from build123d import *

# Parameters (mm, degrees)
EXTRUDE_START               = 15.8125
EXTRUDE_1_OUTLINE_W         = 35.35
EXTRUDE_1_OUTLINE_H         = 28.3375
EXTRUDE_1_DEPTH             = 9.5875
SKETCH_2_W                  = 35.35
SKETCH_2_H                  = 12.7
EXTRUDE_2_DEPTH             = 15.8125
SKETCH_3_W                  = 48.05
SKETCH_3_H                  = 25.4
EXTRUDE_3_DEPTH             = 6.35
SKETCH_4_W                  = 5.925
SKETCH_4_H                  = 6.096
EXTRUDE_4_DEPTH             = 11.5
SKETCH_5_W                  = 5.925
SKETCH_5_H                  = 6.096
EXTRUDE_5_DEPTH             = 11.5
HOLE_WIZARD_1_D             = 3.6576
HOLE_WIZARD_1_DEPTH         = 46.1875
HOLE_WIZARD_2_D             = 3.6576
HOLE_WIZARD_M8_1_D          = 9.525
HOLE_WIZARD_3_D             = 12.7
HOLE_WIZARD_M1_6_1_D        = 1.778
HOLE_WIZARD_M1_6_1_DEPTH    = 6.440714286
HOLE_WIZARD_M1_6_1_TIP      = 0.53416509
HOLE_WIZARD_1_7_1_7_1_D     = 1.7
HOLE_WIZARD_1_7_1_7_1_DEPTH = 9.5875
HOLE_WIZARD_1_5_1_5_1_D     = 1.5
HOLE_WIZARD_1_5_1_5_1_DEPTH = 21.9085


with BuildPart() as part:
    # 凸台-拉伸1: read off the stored shape, not the designer's step
    # 凸台-拉伸1 outline → 凸台-拉伸1 (new body)
    with BuildSketch(Plane(origin=(0, 0, 0), x_dir=(1, 0, 0), z_dir=(0, 1, 0)).offset(EXTRUDE_START)):
        with Locations((6.7, 10.99375)):
            Rectangle(EXTRUDE_1_OUTLINE_W, EXTRUDE_1_OUTLINE_H)
        with BuildLine():
            Line((14.85, 9.525), (-1.45, 9.525))
            ThreePointArc((-1.45, 9.525), (-7.8, 15.875), (-1.45, 22.225))
            Line((-1.45, 22.225), (14.85, 22.225))
            ThreePointArc((14.85, 22.225), (21.2, 15.875), (14.85, 9.525))
        make_face(mode=Mode.SUBTRACT)
    extrude(amount=EXTRUDE_1_DEPTH)

    # 草图2 → 凸台-拉伸2 (add)
    with BuildSketch(Plane.XZ.offset(-15.8125)):
        with Locations((6.7, -3.175)):
            Rectangle(SKETCH_2_W, SKETCH_2_H)
    extrude(amount=EXTRUDE_2_DEPTH)

    # 草图3 → 凸台-拉伸3 (add)
    with BuildSketch(Plane.XY.offset(3.175)):
        with Locations((6.7, 12.7)):
            Rectangle(SKETCH_3_W, SKETCH_3_H)
    extrude(amount=EXTRUDE_3_DEPTH)

    # 草图4 → 凸台-拉伸4 (add)
    with BuildSketch(Plane(origin=(0, 0, -25.1625), x_dir=(-1, 0, 0), z_dir=(0, 0, -1))):
        with Locations((-21.4125, 18.8605)):
            Rectangle(SKETCH_4_W, SKETCH_4_H)
    extrude(amount=EXTRUDE_4_DEPTH)

    # 草图5 → 凸台-拉伸5 (add)
    with BuildSketch(Plane(origin=(0, 0, -25.1625), x_dir=(-1, 0, 0), z_dir=(0, 0, -1))):
        with Locations((8.0125, 18.8605)):
            Rectangle(SKETCH_5_W, SKETCH_5_H)
    extrude(amount=EXTRUDE_5_DEPTH)

    # 孔1
    with Locations(Plane.XY.offset(9.525)):
        with Locations((27.55, 22.225), (27.55, 3.175)):
            Hole(HOLE_WIZARD_1_D / 2, depth=HOLE_WIZARD_1_DEPTH)

    # 孔2 (through all)
    with Locations(Plane(origin=(0, 0, 3.175), x_dir=(-1, 0, 0), z_dir=(0, 0, -1))):
        with Locations((14.15, 3.175), (14.15, 22.225)):
            Hole(HOLE_WIZARD_2_D / 2)

    # M8 间隙孔1 (through all)
    with Locations(Plane(origin=(0, 25.4, 0), x_dir=(1, 0, 0), z_dir=(0, 1, 0))):
        with Locations((0, 0)):
            Hole(HOLE_WIZARD_M8_1_D / 2)

    # 孔3 (through all)
    with Locations(Plane(origin=(0, 0, 0), x_dir=(-1, 0, 0), z_dir=(0, -1, 0))):
        with Locations((-15.875, 0)):
            Hole(HOLE_WIZARD_3_D / 2)

    # M1.6 间隙孔1
    with Locations(Plane(origin=(0, 0, 0), x_dir=(-1, 0, 0), z_dir=(0, -1, 0))):
        with Locations((9.705, -6.35), (8.475, 6.525), (-21.875, 6.525), (-23.105, -6.35)):
            Hole(HOLE_WIZARD_M1_6_1_D / 2, depth=HOLE_WIZARD_M1_6_1_DEPTH)
            with Locations((0, 0, -(HOLE_WIZARD_M1_6_1_DEPTH + HOLE_WIZARD_M1_6_1_TIP / 2))):  # 118° drill point
                Cone(0, HOLE_WIZARD_M1_6_1_D / 2, HOLE_WIZARD_M1_6_1_TIP, mode=Mode.SUBTRACT)

    # Ø1.7 (1.7) 直径孔1
    with Locations(Plane(origin=(0, 15.8125, 0), x_dir=(-1, 0, 0), z_dir=(0, -1, 0))):
        with Locations((-20, 30.1625), (6.6, 30.1625)):
            Hole(HOLE_WIZARD_1_7_1_7_1_D / 2, depth=HOLE_WIZARD_1_7_1_7_1_DEPTH)

    # Ø1.5 (1.5) 直径孔1
    with Locations(Plane(origin=(0, 21.9085, 0), x_dir=(1, 0, 0), z_dir=(0, 1, 0))):
        with Locations((20, 33.1625), (-6.6, 33.1625)):
            Hole(HOLE_WIZARD_1_5_1_5_1_D / 2, depth=HOLE_WIZARD_1_5_1_5_1_DEPTH)


solid = part.part
Part model, mm, in its own coordinate system. A direction names the side the tool comes from. Coordinates: 2 decimals unless noted, no trailing zeros. Order: outer loops, then holes, each group sorted by start corner. A loop starts at its lowest first (then second) coordinate and runs counter-clockwise, first axis right, second up. Notation, with made-up numbers: M 66.5,13.5 L 102.5,13.5 A17 ccw 102.5,30.5 Z; hole C -30.75,4 d4. An arc over 180 degrees is marked long. Use a Markdown table: item, result.
(1) Flat gauge pins, fed straight in: pin 1 (6 mm diameter, centred on y = 14, z = -13.5, fed in from +X) (3 decimals); pin 2 (4.5 mm diameter, centred on x = -7.5, z = -33, fed in from +Y); pin 3 (5 mm diameter, centred on y = 5, z = -7, fed in from -X) (3 decimals). Where does each tip first touch, or does it go through?
A:
| item | result |
|---|---|
| pin 1 | stops at x = 24.375 |
| pin 2 | stops at y = 21.91 |
| pin 3 | stops at x = -10.975 |
(2) Cut at C-C on y = 14. State how many separate pieces and enclosed holes the cut face has, then the cut area to 3 significant figures.
A:
| item | result |
|---|---|
| separate pieces | 1 |
| enclosed holes | 2 |
| area | 556 mm^2 |
(3) Cut at D-D on z = 0. Write the cut outline in (x, y) (1 decimal).
A:
| item | result |
|---|---|
| outline | M -11,0 L -4.8,0 L -4.8,25.4 L -11,25.4 Z; M 4.8,0 L 9.5,0 L 9.5,25.4 L 4.8,25.4 Z; M 22.2,0 L 24.4,0 L 24.4,25.4 L 22.2,25.4 Z |
(4) Tool access for faces 1 (the cylindrical face through (-8.884, 3.265, 6.69)), 2 (the cylindrical face through (-7.8, 20.54, -15.74)), 3 (the flat face through (28, 13, 3.175)), 4 (the flat face through (-8, 21.908, -31)): list every direction of +Z, -Z, +X, -X, +Y, -Y with a clear straight run to the whole face (end or side of a thin tool).
A:
| item | result |
|---|---|
| face 1 | -Y |
| face 2 | +Y, -Y |
| face 3 | -Z, +X, +Y, -Y |
| face 4 | -Z, +X, -X, +Y |
(5) Probe L1, parallel to Y at x = -14, z = 8; L2, parallel to X at y = 7.5, z = -4 (3 decimals). List the from-to ranges inside material, lowest first.
A:
| item | result |
|---|---|
| L1 | y = 0 to 1.35, 5 to 20.4, 24.05 to 25.4 |
| L2 | x = -10.975 to -2.585, 2.585 to 10.943, 20.807 to 24.375 |
(6) Cut at B-B on x = 27.55. Write the cut outline in (y, z) (3 decimals).
A:
| item | result |
|---|---|
| outline | M 0,3.175 L 1.346,3.175 L 1.346,9.525 L 0,9.525 Z; M 5.004,3.175 L 20.396,3.175 L 20.396,9.525 L 5.004,9.525 Z; M 24.054,3.175 L 25.4,3.175 L 25.4,9.525 L 24.054,9.525 Z |
(7) Pull direction X, two halves, no side cores. Call faces 5 (the cylindrical face through (3.78, 12.52, 2.9)), 6 (the flat face through (21, 21.908, -31)), 7 (the conical face through (-9.591, 6.882, 6.246)), 8 (the flat face through (30.725, 13, 6)): released by +X, released by -X, zero draft, split by the parting line, or undercut.
A:
| item | result |
|---|---|
| face 5 | undercut |
| face 6 | zero draft |
| face 7 | undercut |
| face 8 | released by +X |
